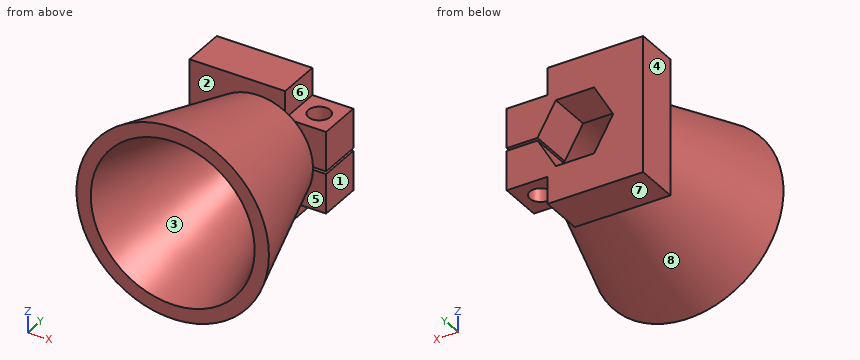
```python
from build123d import *

# Parameters (mm, degrees)
SKETCH2_W                      = 50
SKETCH2_H                      = 50
BOSS_EXTRUDE1_DEPTH            = 16
SKETCH9_W                      = 15
SKETCH9_H                      = 16
CUT_EXTRUDE2_DEPTH             = 10
CBORE_FOR_M4_SHCS2_D           = 5
CBORE_FOR_M4_SHCS2_CBORE_D     = 8
CBORE_FOR_M4_SHCS2_CBORE_DEPTH = 8
SKETCH13_W                     = 15
SKETCH13_H                     = 16
CUT_EXTRUDE5_DEPTH             = 0.5


# Read off the part's stored shape, not the designer's step: Loft-Thin1
with BuildPart() as part:
    # Sketch2 → Boss-Extrude1 (new body)
    with BuildSketch(Plane(origin=(0, 0, 0), x_dir=(1, 0, 0), z_dir=(0, 1, 0))):
        Rectangle(SKETCH2_W, SKETCH2_H)
        Polygon((14, 0), (7, 12.124355653), (-7, 12.124355653), (-14, 0), (-7, -12.124355653), (7, -12.124355653), align=None, mode=Mode.SUBTRACT)
    extrude(amount=BOSS_EXTRUDE1_DEPTH)

    # Loft-Thin1 outline → Loft-Thin1 (revolve)
    with BuildSketch(Plane.XY):
        Polygon((30, -50), (35.220153254, -50), (20.220153254, 0), (15, 0), align=None)
    revolve(axis=Axis((0, 0, 0), (0, 1, 0)))

    # Sketch9 → Cut-Extrude2 (cut)
    with BuildSketch(Plane.XY.offset(25)):
        with Locations((17.5, 8)):
            Rectangle(SKETCH9_W, SKETCH9_H)
    cut_extrude2 = extrude(amount=-CUT_EXTRUDE2_DEPTH, mode=Mode.SUBTRACT)

    # Mirror2: Cut-Extrude2 across plane
    add(cut_extrude2.mirror(Plane.XY), mode=Mode.SUBTRACT)

    # CBORE for M4 SHCS2 (through all)
    with Locations(Plane(origin=(17.5, 8, 15), x_dir=(1, 0, 0), z_dir=(0, 0, 1))):
        with Locations((0, 0)):
            cbore_for_m4_shcs2 = CounterBoreHole(CBORE_FOR_M4_SHCS2_D / 2, CBORE_FOR_M4_SHCS2_CBORE_D / 2, CBORE_FOR_M4_SHCS2_CBORE_DEPTH)

    # Mirror3: CBORE for M4 SHCS2 across plane
    add(cbore_for_m4_shcs2.mirror(Plane.XY), mode=Mode.SUBTRACT)

    # Sketch13 → Cut-Extrude5 (cut, symmetric)
    with BuildSketch(Plane.XY):
        with Locations((17.5, 8)):
            Rectangle(SKETCH13_W, SKETCH13_H)
    extrude(amount=CUT_EXTRUDE5_DEPTH, both=True, mode=Mode.SUBTRACT)


solid = part.part
```
Geometry: final body of the model. Coordinates: model frame, mm. Face numbers are marked on the shaded views. A direction names the side the tool comes from. Coordinates: 2 decimals unless noted, no trailing zeros. Loops run counter-clockwise (first coordinate to the right, second up) from the corner with the lowest first, then second, coordinate; pieces in that order, holes last. Notation, with made-up numbers: (-7, 5.25) -> (52, 5.25) arc R15 cw to (52, 20.25) -> close; hole circle Ø7 at (-26.5, -33.5). An arc over 180 degrees is marked (long way). Use a Markdown table: item, result. Add a question column.
(1) Pin query (flat end, axial travel): pin 1 Ø1.5 at (x, y) = (15.5, 3) entering from -Z; pin 2 Ø3 at (x, y) = (17.5, 8) entering from +Z; pin 3 Ø8 at (y, z) = (8.5, -20) entering from +X; pin 4 Ø4.5 at (y, z) = (7.5, 6) entering from +X. Return the tip coordinate at first contact, or that it passes through.
(2) Section query D-D, the plane y = -20. Return loops of the section in (x, z), plus the area to 3 significant figures.
(3) Section query B-B, the plane x = 0. Return loops of the section in (y, z).
(4) Access query for the marked faces 4, 5, 6, 7 and 8. Directions: +Z, -Z, +X, -X, +Y, -Y. A direction counts if a zero-diameter tool reaches every point of the face in a straight line with its end or side. Return the directions, or none.
(5) Section query A-A, the plane y = 8. State how many separate pieces and enclosed holes the cut face has, plus the area to 3 significant figures.
(6) Mould query, pull axis X, two halves, no side actions, for the marked faces 1, 2 and 3. Classes: pulls with the +X half, pulls with the -X half, needs draft (parallel to the pull), parting line crosses it, or undercut.
(7) Line query: line 1 along Z through (x, y) = (-6.5, 4.5); line 2 along X through (y, z) = (8, -9); line 3 along X through (y, z) = (3, 22). Output: solid intervals per line, ascending.
Answer:
| question | item | result |
|---|---|---|
| 1 | pin 1 | stops at z = -15 |
| 1 | pin 2 | passes through |
| 1 | pin 3 | stops at x = 10 |
| 1 | pin 4 | stops at x = 25 |
| 2 | outline | circle Ø52.44 at (0, 0); hole circle Ø42 at (0, 0) |
| 2 | area | 774 mm^2 |
| 3 | outline | (-50, -35.22) -> (0, -20.22) -> (0, -25) -> (16, -25) -> (16, -12.12) -> (0, -12.12) -> (0, -15) -> (-50, -30) -> close; (-50, 30) -> (0, 15) -> (0, 12.12) -> (16, 12.12) -> (16, 25) -> (0, 25) -> (0, 20.22) -> (-50, 35.22) -> close |
| 4 | face 4 | +Z, -Z, -X, +Y |
| 4 | face 5 | -Z, +X |
| 4 | face 6 | +Z, +X, +Y |
| 4 | face 7 | -Z, +X, -X, +Y |
| 4 | face 8 | none |
| 5 | separate pieces | 3 |
| 5 | enclosed holes | 0 |
| 5 | area | 1,490 mm^2 |
| 6 | face 1 | pulls with the +X half |
| 6 | face 2 | needs draft |
| 6 | face 3 | undercut |
| 7 | line 1 | z = -25 to -12.12, 12.12 to 25 |
| 7 | line 2 | x = -25 to -8.8, 8.8 to 13.5, 21.5 to 25 |
| 7 | line 3 | x = -25 to 10 |
